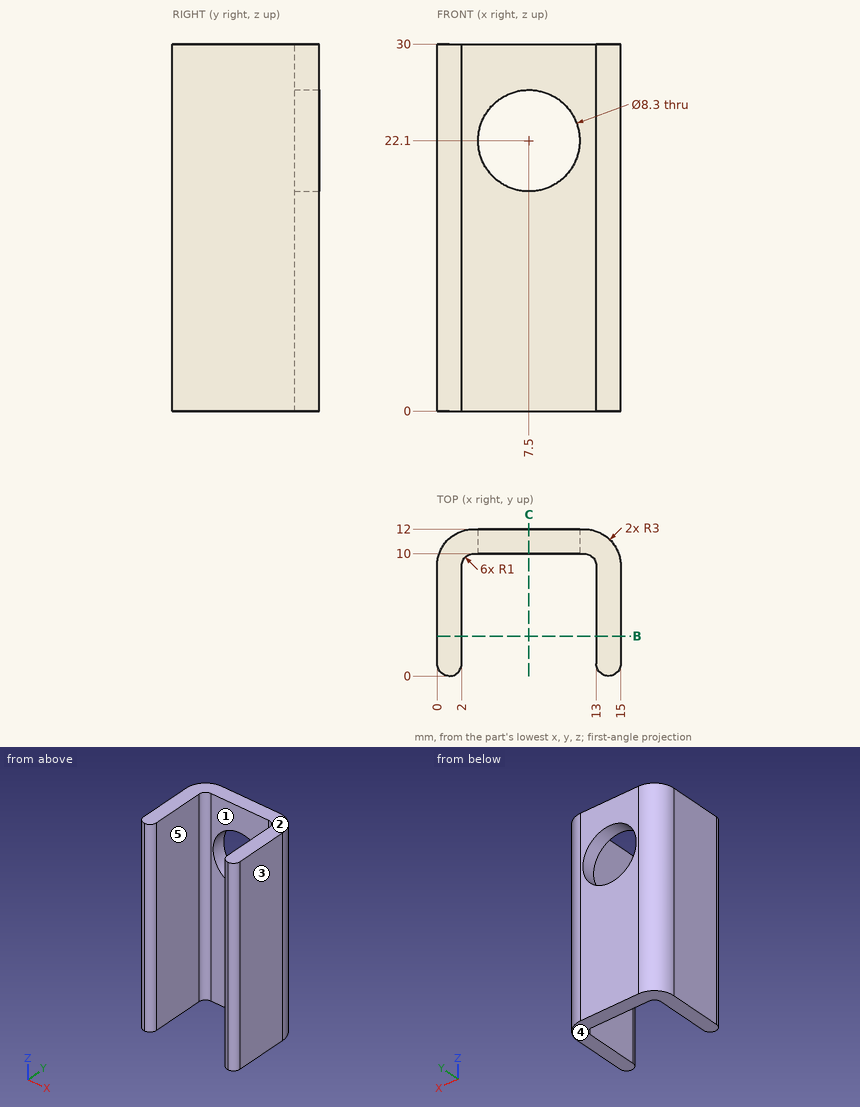
Drawing for the job (mm, zero at the part's lowest x, y, z). A direction names the side the tool comes from. Round coordinates to 2 decimals unless told otherwise and drop trailing zeros. Write each loop counter-clockwise with the first axis right and the second up, starting at its lowest first coordinate (ties: lowest second). Pieces come first, ordered by that corner, then holes.
Item 1: Drop flat-ended pins along their axis: pin 1 Ø2.5 at (x, z) = (6.5, 16.5) entering from -Y; pin 2 Ø7.5 at (x, z) = (7.5, 22.1) entering from -Y. Give the stop position or say it passes through.
Filled in:
pin 1: stops at y = 10
pin 2: passes through
Item 2: Mould opens along X. For the marked faces 1, 2 and 3 say: released by +X, released by -X, zero draft, split by the parting line, or undercut.
Filled in:
face 1: undercut
face 2: zero draft
face 3: released by +X
Item 3: Band-saw the part on C-C on x = 7.5. Write the cut outline in (y, z).
Filled in:
outline: (10, 0) - (12, 0) - (12, 17.95) - (10, 17.95) - close; (10, 26.25) - (12, 26.25) - (12, 30) - (10, 30) - close
Item 4: Drill centre lines: L1, parallel to X at y = 5, z = 2.75; L2, parallel to Z at x = 7.5, y = 10.5; L3, parallel to Y at x = 11.5, z = 10.5. Where is each one in solid material? Low to high.
Filled in:
L1: x = 0 to 2, 13 to 15
L2: z = 0 to 17.95, 26.25 to 30
L3: y = 10 to 12
Item 5: Tool access for the marked faces 4 and 5: list every direction of +Z, -Z, +X, -X, +Y, -Y with a clear straight run to the whole face (end or side of a thin tool).
Filled in:
face 4: -Z, +X, -X, +Y, -Y
face 5: +Z, -Z, -Y
Item 6: Band-saw the part on B-B on y = 3.25. Write the cut outline in (x, z), then the cut area to 3 significant figures.
Filled in:
outline: (0, 0) - (2, 0) - (2, 30) - (0, 30) - close; (13, 0) - (15, 0) - (15, 30) - (13, 30) - close
area: 120 mm2
